from build123d import *

# Parameters (mm, degrees)
EXTRUDE_1_DEPTH     = 5.33
SKETCH_1_W          = 0.5
SKETCH_1_H          = 0.5
EXTRUDE_2_DEPTH     = 2.54
SKETCH_1_2_W        = 0.5
SKETCH_1_2_H        = 0.5
EXTRUDE_3_DEPTH     = 10.16
SKETCH_4_R          = 0.2
CUT_EXTRUDE_1_DEPTH = 0.5
SKETCH_5_W          = 0.5
SKETCH_5_H          = 10.2
EXTRUDE_4_DEPTH     = 2.5
SKETCH_6_W          = 10.2
SKETCH_6_H          = 0.5
EXTRUDE_5_DEPTH     = 2.5
SKETCH_7_W          = 10.2
SKETCH_7_H          = 0.5
EXTRUDE_6_DEPTH     = 2.5
FILLET_1_R          = 2.5
FILLET_2_R          = 1
CUT_EXTRUDE_2_DEPTH = 2.5
CUT_EXTRUDE_3_DEPTH = 1
SKETCH_11_W         = 10.061772152
SKETCH_11_H         = 6.60723038
CUT_EXTRUDE_4_DEPTH = 5.5
SKETCH_12_R         = 0.156456915
CUT_EXTRUDE_5_DEPTH = 1


with BuildPart() as part:
    # Эскиз3 → Вытянуть1 (new body)
    with BuildSketch(Plane.XY.offset(2.54)):
        with BuildLine():
            Line((-0.325, -1.53), (3.105, -1.53))
            Line((3.105, -1.53), (3.99, 0))
            ThreePointArc((3.99, 0), (3.240904038, 1.868477631), (1.39, 2.66))
            ThreePointArc((1.39, 2.66), (-0.460904038, 1.868477631), (-1.21, 0))
            Line((-1.21, 0), (-0.325, -1.53))
        make_face()
    extrude(amount=EXTRUDE_1_DEPTH)

    # Эскиз1 → Вытянуть2 (add)
    with BuildSketch(Plane.XY):
        with Locations((1.39, 0)):
            Rectangle(SKETCH_1_W, SKETCH_1_H)
        Rectangle(SKETCH_1_W, SKETCH_1_H)
        with Locations((2.78, 0)):
            Rectangle(SKETCH_1_W, SKETCH_1_H)
    extrude(amount=EXTRUDE_2_DEPTH)

    # Эскиз1<2> → Вытянуть3 (add)
    with BuildSketch(Plane.XY):
        with Locations((1.39, 0)):
            Rectangle(SKETCH_1_2_W, SKETCH_1_2_H)
        Rectangle(SKETCH_1_2_W, SKETCH_1_2_H)
        with Locations((2.78, 0)):
            Rectangle(SKETCH_1_2_W, SKETCH_1_2_H)
    extrude(amount=-EXTRUDE_3_DEPTH)

    # Эскиз4 → Вырез-Вытянуть1 (cut)
    with BuildSketch(Plane.XY.offset(7.87)):
        Circle(SKETCH_4_R)
    extrude(amount=-CUT_EXTRUDE_1_DEPTH, mode=Mode.SUBTRACT)

    # Эскиз5 → Вытянуть4 (add)
    with BuildSketch(Plane(origin=(0, -0.25, 0), x_dir=(1, 0, 0), z_dir=(0, 1, 0))):
        with Locations((1.39, 5.06)):
            Rectangle(SKETCH_5_W, SKETCH_5_H)
    extrude(amount=-EXTRUDE_4_DEPTH)

    # Эскиз6 → Вытянуть5 (add)
    with BuildSketch(Plane.ZY.offset(0.25)):
        with Locations((-5.06, 0)):
            Rectangle(SKETCH_6_W, SKETCH_6_H)
    extrude(amount=EXTRUDE_5_DEPTH)

    # Эскиз7 → Вытянуть6 (add)
    with BuildSketch(Plane(origin=(3.03, 0, 0), x_dir=(0, 0, -1), z_dir=(1, 0, 0))):
        with Locations((5.06, 0)):
            Rectangle(SKETCH_7_W, SKETCH_7_H)
    extrude(amount=EXTRUDE_6_DEPTH)

    # Скругление1
    fillet_1_edges = [part.edges().sort_by_distance(p)[0] for p in [
        (5.53, 0, 0.04),
        (-2.75, 0, 0.04),
        (1.39, -2.75, 0.04),
    ]]
    fillet(fillet_1_edges, radius=FILLET_1_R - 0.0001)  # a hair under: the kernel refuses the full size

    # Скругление2
    fillet_2_edges = [part.edges().sort_by_distance(p)[0] for p in [
        (-0.25, 0, 0.04),
        (3.03, 0, 0.04),
        (1.39, -0.25, 0.04),
    ]]
    fillet(fillet_2_edges, radius=FILLET_2_R)

    # Эскиз9 → Вырез-Вытянуть2 (cut)
    with BuildSketch(Plane.XZ.offset(0.25)):
        with BuildLine():
            Line((-2.25, -10.16), (-2.25, -2.46))
            ThreePointArc((-2.25, -2.46), (-1.853567451, -1.264771391), (-0.821428571, -0.543370305))
            ThreePointArc((-0.821428571, -0.543370305), (-0.047324411, -0.002319491), (0.25, 0.894101966))
            Line((0.25, 0.894101966), (0.25, -10.16))
            Line((0.25, -10.16), (-2.25, -10.16))
        make_face()
        with BuildLine():
            Line((5.03, -10.16), (2.53, -10.16))
            Line((2.53, -10.16), (2.53, 0.894101966))
            ThreePointArc((2.53, 0.894101966), (2.827324411, -0.002319491), (3.601428571, -0.543370305))
            ThreePointArc((3.601428571, -0.543370305), (4.633567451, -1.264771391), (5.03, -2.46))
            Line((5.03, -2.46), (5.03, -10.16))
        make_face()
    extrude(amount=-CUT_EXTRUDE_2_DEPTH, mode=Mode.SUBTRACT)

    # Эскиз10 → Вырез-Вытянуть3 (cut)
    with BuildSketch(Plane.ZY.offset(-1.14)):
        with BuildLine():
            Line((-2.46, -2.25), (-10.16, -2.25))
            Line((-10.16, -2.25), (-10.16, 0.25))
            Line((-10.16, 0.25), (0.894101966, 0.25))
            ThreePointArc((0.894101966, 0.25), (-0.002319491, -0.047324411), (-0.543370305, -0.821428571))
            ThreePointArc((-0.543370305, -0.821428571), (-1.264771391, -1.853567451), (-2.46, -2.25))
        make_face()
    extrude(amount=-CUT_EXTRUDE_3_DEPTH, mode=Mode.SUBTRACT)

    # Эскиз11 → Вырез-Вытянуть4 (cut)
    with BuildSketch(Plane(origin=(0, 0, -10.16), x_dir=(-1, 0, 0), z_dir=(0, 0, -1))):
        with Locations((-1.088146835, -1.646498734)):
            Rectangle(SKETCH_11_W, SKETCH_11_H)
    extrude(amount=-CUT_EXTRUDE_4_DEPTH, mode=Mode.SUBTRACT)

    # Эскиз12 → Вырез-Вытянуть5 (cut)
    with BuildSketch(Plane(origin=(0, 0, -4.66), x_dir=(-1, 0, 0), z_dir=(0, 0, -1))):
        with Locations((-1.39, -2.5)):
            Circle(SKETCH_12_R)
    extrude(amount=-CUT_EXTRUDE_5_DEPTH, mode=Mode.SUBTRACT)


solid = part.part
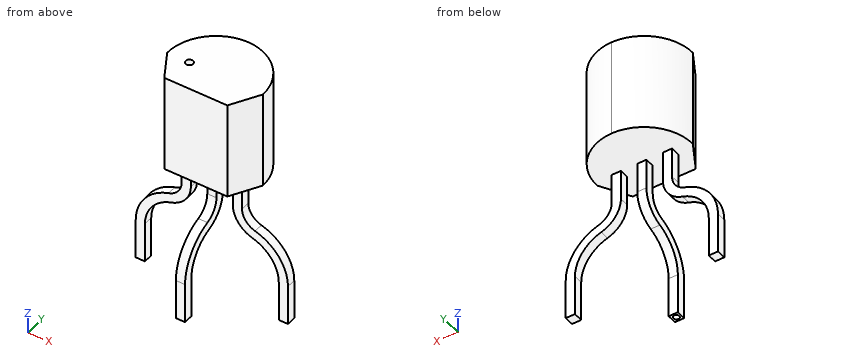
Design review of the part built by this model. Coordinates are the model's own, in mm. Give positions to 0.01 mm unless a question says otherwise; leave off trailing zeros. Write each loop counter-clockwise with the first axis right and the second up, starting at its lowest first coordinate (ties: lowest second). Pieces come first, ordered by that corner, then holes. Notation, with made-up numbers: M -4,25.5 L 23,25.5 A29 ccw 23,60.5 Z; hole C 73,48.25 d7. An arc over 180 degrees is marked long. Return JSON: item names as keys, results as strings. Group by question number.
Item 1: Take a section at A-A (z = 1.25). Give the boundary of the cut face in (x, y).
Item 2: Take a section at B-B (y = -1.35). Give the boundary of the cut face in (x, z), plus the area to 3 significant figures.
Item 3: Take a section at D-D (y = -2.5). Give the boundary of the cut face in (x, z), plus the area to 3 significant figures.
Item 4: Wall thickness on line 1 along Z through (x, y) = (2.75, -1.35); line 2 along X through (y, z) = (-2.35, -2); line 3 along Y through (x, z) = (0, 7.7): over which ranges is each line inside the solid? List them lowest first.
Item 5: Clearance check with flat-ended pins moving along their axes: pin 1 Ø0.6 at (y, z) = (0, 1.5) entering from -X; pin 2 Ø1.5 at (x, z) = (-0.5, -2) entering from +Y; pin 3 Ø1.5 at (x, z) = (4.5, -3) entering from -Y; pin 4 Ø2.5 at (y, z) = (-2, 0) entering from +X. State where each tip first meets the part, or that it passes through.
Item 6: Take a section at C-C (x = 0). Give the boundary of the cut face in (y, z), plus the area to 3 significant figures.
Return value:
{
 "1": {"outline": "M -0.25,-0.25 L 0.25,-0.25 L 0.25,0.25 L -0.25,0.25 Z; M 1.14,-0.25 L 1.64,-0.25 L 1.64,0.25 L 1.14,0.25 Z; M 2.53,-0.25 L 3.03,-0.25 L 3.03,0.25 L 2.53,0.25 Z"},
 "2": {"outline": "M -0.43,2.54 L 3.21,2.54 L 3.21,7.87 L -0.43,7.87 Z; M 1.14,-0.79 L 1.64,-0.79 L 1.64,-0.21 L 1.14,-0.21 Z", "area": "19.7 mm2"},
 "3": {"outline": "M 1.14,-4.66 L 1.23,-4.66 L 1.23,-3.66 L 1.55,-3.66 L 1.55,-4.66 L 1.64,-4.66 L 1.64,-1.37 L 1.14,-1.37 Z", "area": "1.33 mm2"},
 "4": {"line 1": "z = 2.54 to 7.87", "line 2": "x = 1.14 to 1.64", "line 3": "y = -1.53 to -0.2, 0.2 to 2.24"},
 "5": {"pin 1": "stops at x = -0.25", "pin 2": "passes through", "pin 3": "stops at y = -0.25", "pin 4": "stops at x = 1.64"},
 "6": {"outline": "M -1.53,2.54 L -0.25,2.54 L -0.25,0.06 L 0.25,0.06 L 0.25,2.54 L 2.24,2.54 L 2.24,7.87 L 0.2,7.87 L 0.2,7.37 L -0.2,7.37 L -0.2,7.87 L -1.53,7.87 Z", "area": "21.2 mm2"}
}
